The figure shows three views and two pictorial views of one solid part (mm, origin at its lowest corner). Answer the questions. Round coordinates to 2 decimals unless told otherwise and drop trailing zeros. Order: outer loops, then holes, each group sorted by start corner. A loop starts at its lowest first (then second) coordinate and runs counter-clockwise, first axis right, second up. Notation, with made-up numbers: M -11.5,-30.5 L 14.5,-30.5 A35 cw 14.5,5.5 Z; hole C 73,-11.75 d4. An arc over 180 degrees is marked long. Return JSON: item names as keys, results as strings.
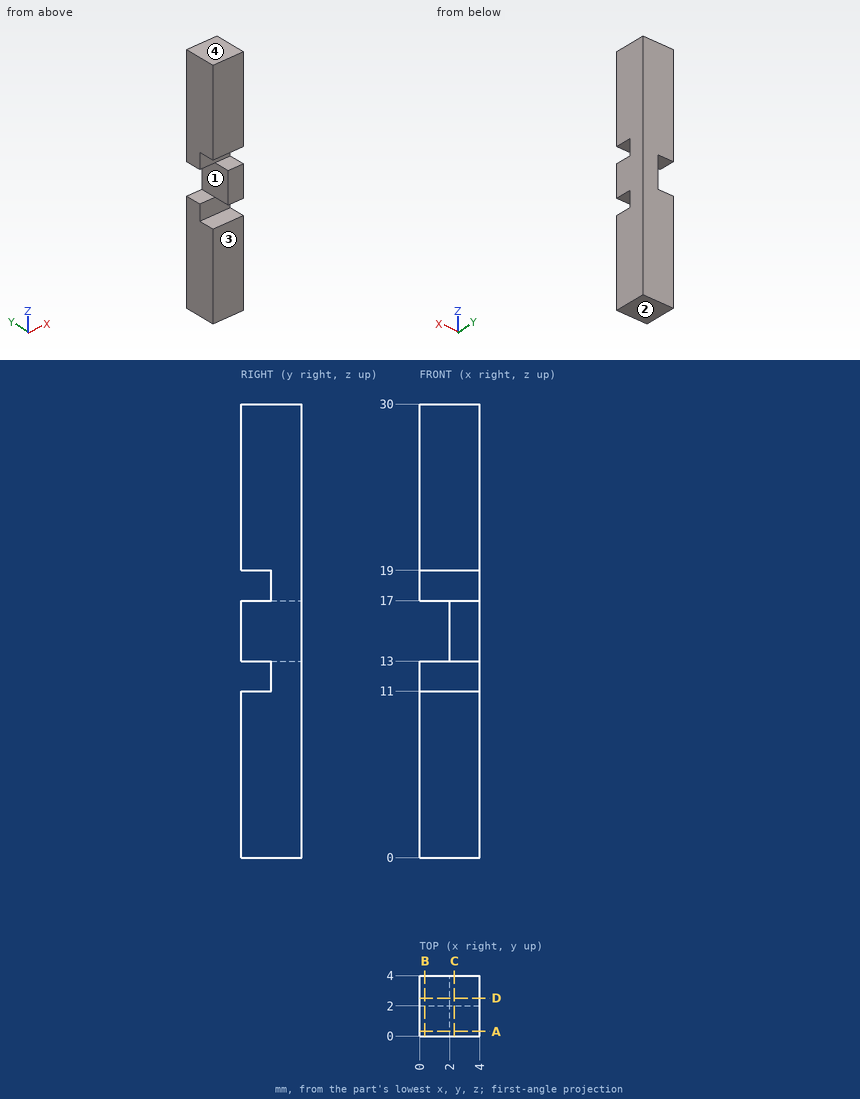
Item 1: Consider line 1 along Z through (x, y) = (1.9, 1.95); line 2 along Y through (x, z) = (2.4, 18.5). Determine where each line is inside the solid, lowest interval first. Write a range as [from, to].
Output:
{"line 1": "z = [0, 11], [19, 30]", "line 2": "y = [2, 4]"}
Item 2: Find section A-A (y = 0.3). Determine the outline of the cut face in (x, z).
Output:
{"outline": "M 0,0 L 4,0 L 4,11 L 0,11 Z; M 0,19 L 4,19 L 4,30 L 0,30 Z; M 2,13 L 4,13 L 4,17 L 2,17 Z"}
Item 3: Find section D-D (y = 2.5). Determine the outline of the cut face in (x, z), plus the area to 3 significant figures.
Output:
{"outline": "M 0,0 L 4,0 L 4,30 L 0,30 L 0,17 L 2,17 L 2,13 L 0,13 Z", "area": "112 mm^2"}
Item 4: Find section C-C (x = 2.3). Determine the outline of the cut face in (y, z).
Output:
{"outline": "M 0,0 L 4,0 L 4,30 L 0,30 L 0,19 L 2,19 L 2,17 L 0,17 L 0,13 L 2,13 L 2,11 L 0,11 Z"}
Item 5: The mould has two halves that part along Z. Classify the marked faces 1, 2, 3 and 4: pulls with the +Z half, pulls with the -Z half, needs draft (parallel to the pull), parting line crosses it, or undercut.
Output:
{"face 1": "undercut", "face 2": "pulls with the -Z half", "face 3": "needs draft", "face 4": "pulls with the +Z half"}
Item 6: Each of these flat-tipped pins is pushed along its axis until it touches: pin 1 (0.6 mm diameter, centred on x = 2, y = 0.5, fed in from -Z); pin 2 (1 mm diameter, centred on x = 1.5, z = 12, fed in from -Y). Where does it stop, or does it pass through?
Output:
{"pin 1": "stops at z = 0", "pin 2": "stops at y = 2"}
Item 7: Find section B-B (x = 0.35). Determine the outline of the cut face in (y, z), plus the area to 3 significant figures.
Output:
{"outline": "M 0,0 L 4,0 L 4,13 L 2,13 L 2,11 L 0,11 Z; M 0,19 L 2,19 L 2,17 L 4,17 L 4,30 L 0,30 Z", "area": "96.0 mm^2"}
